from build123d import *

# Parameters (mm, degrees)
F0_W     = 45
F0_H     = 26
F1_DEPTH = 26
F2_W     = 24
F2_H     = 24
F3_DEPTH = 45.001
F5_D     = 4.4
F7_D     = 4.4


with BuildPart() as f1:
    # F0 (on Top) → F1 (new body)
    with BuildSketch(Plane.XY):
        with Locations((-10.5, 0)):
            Rectangle(F0_W, F0_H)
    extrude(amount=F1_DEPTH)

    # F2 (on face) → F3 (cut, through all)
    with BuildSketch(Plane.YZ.offset(12)):
        with Locations((-1, 14)):
            Rectangle(F2_W, F2_H)
    extrude(amount=-F3_DEPTH, mode=Mode.SUBTRACT)

    # F5 (through all)
    with Locations(Plane.XY.offset(2)):
        with Locations((0, 0), (3, -9)):
            Hole(F5_D / 2)

    # F7 (through all)
    with Locations(Plane.XZ.offset(-11)):
        with Locations((-29, 19), (8, 19)):
            Hole(F7_D / 2)


solid = f1.part
Here's how the part is built. I have some questions about the finished solid (model axes, mm). A direction names the side the tool comes from. Coordinates: 2 decimals unless noted, no trailing zeros. Write each loop counter-clockwise with the first axis right and the second up, starting at its lowest first coordinate (ties: lowest second). Pieces come first, ordered by that corner, then holes.
Item 1: If we mould it in two halves opening along Z, with no side actions, what happens to faces 1 (the flat face through (-10, -1, 2)), 2 (the flat face through (-33, 6, 1)), 3 (the cylindrical face through (-27.254, 12.014, 17.661))? For each: +Z half, -Z half, draft (parallel to the pull), parting line (faces both ways), or undercut.
Item 2: Will these pins go through, and if not, where does the flat tip stop? pin 1 (1.5 mm diameter, centred on x = -27, y = 10, fed in from +Z); pin 2 (2.5 mm diameter, centred on x = 0, y = 0, fed in from -Z); pin 3 (1 mm diameter, centred on x = -5, z = 11, fed in from -Y); pin 4 (12 mm diameter, centred on x = 2.5, y = 10, fed in from +Z).
Item 3: I want a section at A-A on z = 19. Write out the boundary of the cut face in (x, y), and give its area (3 significant figures).
Item 4: If I drill on line 1 (Y direction, x = -20.5, z = 14.25); line 2 (Y direction, x = 0, z = 1.5); line 3 (Z direction, x = -29, y = 12.05), over which ranges is the centre line in solid material (lowest first)?
Item 5: I want a section at C-C on x = 8. Write out the boundary of the cut face in (y, z).
Item 6: I want a section at B-B on y = -9. Write out the boundary of the cut face in (x, z), and give its area (3 significant figures).
Item 7: On a 3-axis mill with a long thin cutter (end or side, diameter ignored), from which of +Z, -Z, +X, -X, +Y, -Y can I reach the whole of each face in a straight line? I mean faces 4 (the flat face through (-10, 11, 14)), 5 (the cylindrical face through (3.29, -6.82, 0.99)). Say none if no direction works.
Item 8: I want a section at D-D on x = -21. Write out the boundary of the cut face in (y, z), and give its area (3 significant figures).
Findings below:
1. face 1: +Z half
1. face 2: draft
1. face 3: undercut
2. pin 1: stops at z = 2
2. pin 2: passes through
2. pin 3: stops at y = 11
2. pin 4: stops at z = 26
3. outline: (-33, 11) - (-31.2, 11) - (-31.2, 13) - (-33, 13) - close; (-26.8, 11) - (5.8, 11) - (5.8, 13) - (-26.8, 13) - close; (10.2, 11) - (12, 11) - (12, 13) - (10.2, 13) - close
3. area: 72.4 mm2
4. line 1: y = 11 to 13
4. line 2: y = -13 to -2.2, 2.2 to 13
4. line 3: z = 0 to 16.8, 21.2 to 26
5. outline: (-13, 0) - (13, 0) - (13, 16.8) - (11, 16.8) - (11, 2) - (-13, 2) - close; (11, 21.2) - (13, 21.2) - (13, 26) - (11, 26) - close
6. outline: (-33, 0) - (0.8, 0) - (0.8, 2) - (-33, 2) - close; (5.2, 0) - (12, 0) - (12, 2) - (5.2, 2) - close
6. area: 81.2 mm2
7. face 4: +Z, +X, -X, -Y
7. face 5: +Z, -Z
8. outline: (-13, 0) - (13, 0) - (13, 26) - (11, 26) - (11, 2) - (-13, 2) - close
8. area: 100 mm2
